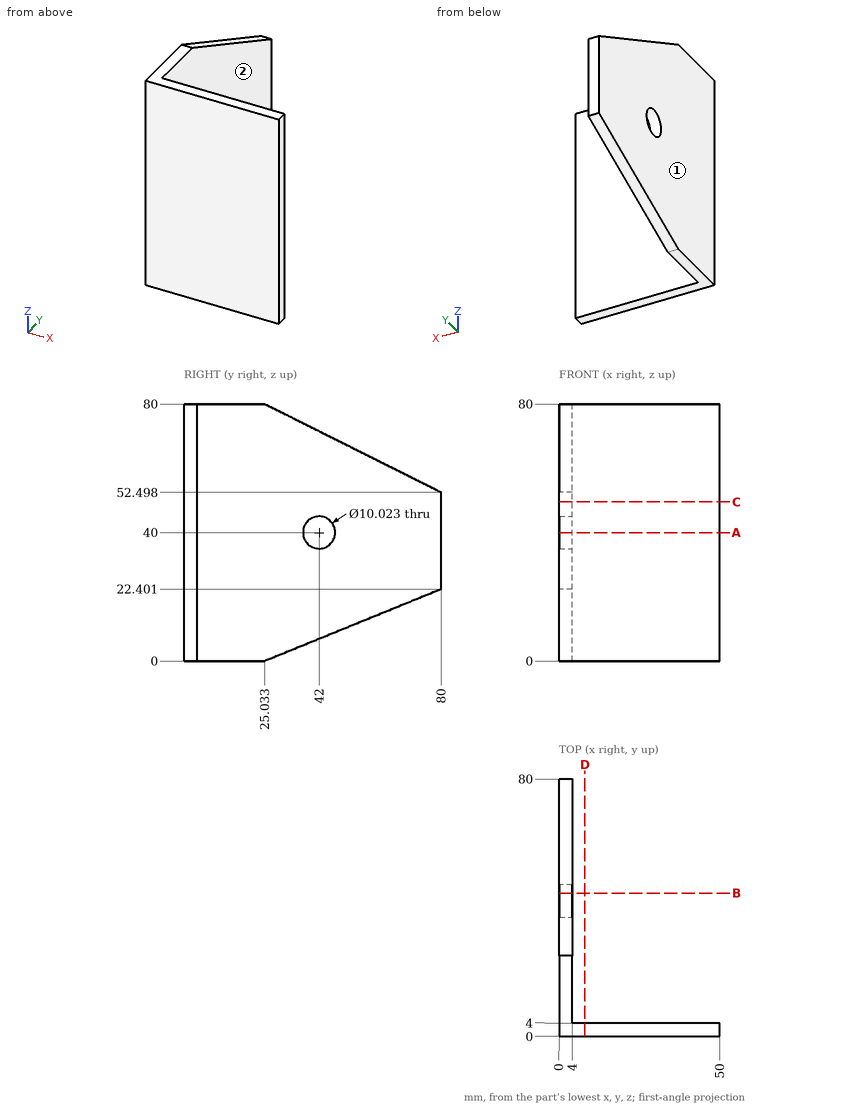
Geometry check sheet. Reference: drawing and pictorial views, mm from the part's lowest x, y, z. A direction names the side the tool comes from. Coordinates: 2 decimals unless noted, no trailing zeros. Order: outer loops, then holes, each group sorted by start corner. A loop starts at its lowest first (then second) coordinate and runs counter-clockwise, first axis right, second up. Notation, with made-up numbers: (21, 15) - (64, 15) arc R19 ccw to (64, 38) - close; hole circle Ø2 at (5.5, 42.5). An arc over 180 degrees is marked (long way). Answer in a Markdown table with one row per item. Add a question column.
1) Material ranges on line 1 along Y through (x, z) = (15, 51); line 2 along Z through (x, y) = (1, 42) (1 decimal), recorded low to high. Write a range as [from, to].
2) Cross-section at C-C, the plane z = 49.5. Record the cut outline in (x, y), then the cut area to 3 significant figures.
3) Cross-section at D-D, the plane x = 8. Record the cut outline in (y, z).
4) Cross-section at A-A, the plane z = 40. Record the cut outline in (x, y), then the cut area to 3 significant figures.
5) Set-up check for the marked faces 1 and 2: record each of +Z, -Z, +X, -X, +Y, -Y from which the full face is reachable in a straight line by a thin tool's end or side.
6) Cross-section at B-B, the plane y = 44.5. Record the cut outline in (x, z).
7) Gauge pin test, flat ends, axial feed: P1, Ø1, axis at x = 41.5, z = 66.5, coming from the +Y side; P2, Ø5, axis at y = 41, z = 58.5, coming from the +X side; P3, Ø10, axis at y = 13.5, z = 45.5, coming from the -X side. Record the tip position at first contact, or that the pin passes through.
Check result:
| question | item | result |
|---|---|---|
| 1 | line 1 | y = [0, 4] |
| 1 | line 2 | z = [6.9, 35], [45, 71.5] |
| 2 | outline | (0, 0) - (50, 0) - (50, 4) - (4, 4) - (4, 80) - (0, 80) - close |
| 2 | area | 504 mm² |
| 3 | outline | (0, 0) - (4, 0) - (4, 80) - (0, 80) - close |
| 4 | outline | (0, 0) - (50, 0) - (50, 4) - (4, 4) - (4, 36.99) - (0, 36.99) - close; (0, 47.01) - (4, 47.01) - (4, 80) - (0, 80) - close |
| 4 | area | 464 mm² |
| 5 | face 1 | +Z, -Z, -X, +Y, -Y |
| 5 | face 2 | +Z, -Z, +X, +Y |
| 6 | outline | (0, 7.93) - (4, 7.93) - (4, 35.66) - (0, 35.66) - close; (0, 44.34) - (4, 44.34) - (4, 70.26) - (0, 70.26) - close |
| 7 | P1 | stops at y = 4 |
| 7 | P2 | stops at x = 4 |
| 7 | P3 | stops at x = 0 |
